```python
from build123d import *

# Parameters (mm, degrees)
SKETCH1_R                   = 1.25
SKETCH1_R_2                 = 1.525
BOSS_EXTRUDE1_DEPTH         = 2
SKETCH3_R                   = 2
BOSS_EXTRUDE2_DEPTH         = 8
M3_TAPPED_HOLE1_D           = 2.5
M3_TAPPED_HOLE1_DEPTH       = 6
M3_TAPPED_HOLE1_CSINK_D     = 3.05
M3_TAPPED_HOLE1_CSINK_ANGLE = 90
M3_TAPPED_HOLE1_TIP         = 0.751075774
FILLET1_R                   = 2


with BuildPart() as part:
    # Sketch1 → Boss-Extrude1 (new body)
    with BuildSketch(Plane.XY):
        with BuildLine():
            Line((-37.5, 57.260829493), (37.5, 57.260829493))
            ThreePointArc((37.5, 57.260829493), (41.035533906, 55.796363399), (42.5, 52.260829493))
            Line((42.5, 52.260829493), (42.5, -57.739170507))
            ThreePointArc((42.5, -57.739170507), (41.035533906, -61.274704413), (37.5, -62.739170507))
            Line((37.5, -62.739170507), (-37.5, -62.739170507))
            ThreePointArc((-37.5, -62.739170507), (-41.035533906, -61.274704413), (-42.5, -57.739170507))
            Line((-42.5, -57.739170507), (-42.5, 52.260829493))
            ThreePointArc((-42.5, 52.260829493), (-41.035533906, 55.796363399), (-37.5, 57.260829493))
        make_face()
        with Locations((36.3, -56.539170507)):
            Circle(SKETCH1_R, mode=Mode.SUBTRACT)
        with Locations((36.3, 51.060829493)):
            Circle(SKETCH1_R_2, mode=Mode.SUBTRACT)
        with Locations((-36.3, 51.060829493)):
            Circle(SKETCH1_R_2, mode=Mode.SUBTRACT)
        with Locations((-36.3, -56.539170507)):
            Circle(SKETCH1_R_2, mode=Mode.SUBTRACT)
    extrude(amount=BOSS_EXTRUDE1_DEPTH)

    # Sketch3 → Boss-Extrude2 (add)
    with BuildSketch(Plane(origin=(0, 0, 0), x_dir=(-1, 0, 0), z_dir=(0, 0, -1))):
        with Locations((-19.5, 36.260829493)):
            Circle(SKETCH3_R)
        with Locations((19.5, 36.260829493)):
            Circle(SKETCH3_R)
        with Locations((19.5, -2.739170507)):
            Circle(SKETCH3_R)
        with Locations((-19.5, -2.739170507)):
            Circle(SKETCH3_R)
    extrude(amount=BOSS_EXTRUDE2_DEPTH)

    # M3 Tapped Hole1
    with Locations(Plane(origin=(0, 0, -8), x_dir=(-1, 0, 0), z_dir=(0, 0, -1))):
        with Locations((-19.5, -2.739170507), (-19.5, 36.260829493), (19.5, 36.260829493), (19.5, -2.739170507)):
            CounterSinkHole(M3_TAPPED_HOLE1_D / 2, M3_TAPPED_HOLE1_CSINK_D / 2, depth=M3_TAPPED_HOLE1_DEPTH, counter_sink_angle=M3_TAPPED_HOLE1_CSINK_ANGLE)
            with Locations((0, 0, -(M3_TAPPED_HOLE1_DEPTH + M3_TAPPED_HOLE1_TIP / 2))):  # 118° drill point
                Cone(0, M3_TAPPED_HOLE1_D / 2, M3_TAPPED_HOLE1_TIP, mode=Mode.SUBTRACT)

    # Fillet1
    fillet1_edges = [part.edges().sort_by_distance(p)[0] for p in [
        (21.5, 36.260829493, 0),
        (-17.5, 36.260829493, 0),
        (-17.5, -2.739170507, 0),
        (21.5, -2.739170507, 0),
    ]]
    fillet(fillet1_edges, radius=FILLET1_R)


solid = part.part
```
CAD build for the part. Positions are in the model's coordinates, mm. A direction names the side the tool comes from. Coordinates: 2 decimals unless noted, no trailing zeros. Write each loop counter-clockwise with the first axis right and the second up, starting at its lowest first coordinate (ties: lowest second). Pieces come first, ordered by that corner, then holes.
(1) Drill centre lines: probe 1 along Y at (x, z) = (36.3, 0.85); probe 2 along Y at (x, z) = (19.5, -4.75); probe 3 along Y at (x, z) = (-19, -3.25). Where is each one in solid material? Low to high.
(2) Cut at D-D, the plane y = -43.5. List the corners of the cut face in (x, z).
(3) Cut at C-C, the plane x = 36.3. List the corners of the cut face in (y, z), and give its area (3 significant figures).
(4) Cut at B-B, the plane z = -5. List the corners of the cut face in (x, y), and give its area (3 significant figures).
(5) Two-plate mould, pull along X, no slides. Class faces 3 (the face through (-19.66, 37.5, -4.82)), 4 (the face through (40.996, 55.835, 0.986)): +X half, -X half, draft (parallel to the pull), parting line (faces both ways), or undercut.
(6) Flat gauge pins, fed straight in: pin 1 (1.5 mm diameter, centred on y = 38.5, z = -4.5, fed in from -X); pin 2 (4 mm diameter, centred on x = -36.3, y = -56.54, fed in from -Z). Where does each tip first touch, or does it go through?
(7) 3-axis set-ups, long thin cutter, end or side, ignore diameter. For faces 1 (the face through (21.5, -2.7, -5)), 2 (the face through (41.07, -61.24, 0.99)): which of +Z, -Z, +X, -X, +Y, -Y reach the whole face in a straight line?
(8) Cut at A-A, the plane x = -36.3. List the corners of the cut face in (y, z), and give its area (3 significant figures).
Geometry says:
1. probe 1: y = -62.74 to -57.79, -55.29 to 49.54, 52.59 to 57.26
1. probe 2: y = -4.74 to -3.99, -1.49 to -0.74, 34.26 to 35.01, 37.51 to 38.26
1. probe 3: y = -4.68 to -3.88, -1.59 to -0.8, 34.32 to 35.12, 37.41 to 38.2
2. outline: (-42.5, 0) - (42.5, 0) - (42.5, 2) - (-42.5, 2) - close
3. outline: (-62.74, 0) - (-57.79, 0) - (-57.79, 2) - (-62.74, 2) - close; (-55.29, 0) - (49.54, 0) - (49.54, 2) - (-55.29, 2) - close; (52.59, 0) - (57.26, 0) - (57.26, 2) - (52.59, 2) - close
3. area: 229 mm2
4. outline: circle Ø4 at (-19.5, -2.74); circle Ø4 at (-19.5, 36.26); circle Ø4 at (19.5, -2.74); circle Ø4 at (19.5, 36.26); hole circle Ø2.5 at (-19.5, -2.74); hole circle Ø2.5 at (-19.5, 36.26); hole circle Ø2.5 at (19.5, -2.74); hole circle Ø2.5 at (19.5, 36.26)
4. area: 30.6 mm2
5. face 3: undercut
5. face 4: +X half
6. pin 1: stops at x = -20.84
6. pin 2: stops at z = 0
7. face 1: -Z
7. face 2: +Z, -Z, +X, -Y
8. outline: (-62.74, 0) - (-58.06, 0) - (-58.06, 2) - (-62.74, 2) - close; (-55.01, 0) - (49.54, 0) - (49.54, 2) - (-55.01, 2) - close; (52.59, 0) - (57.26, 0) - (57.26, 2) - (52.59, 2) - close
8. area: 228 mm2
